Autodesk Inventor part; units mm, degrees
sketch "Sketch1" plane through (0, 0, 0) normal (0, 0, 1) x (1, 0, 0)
  line L0 (-10.75, -9.35) -> (10.75, -9.35)
  line L1 (10.75, -9.35) -> (10.75, 9.35)
  line L2 (10.75, 9.35) -> (-10.75, 9.35)
  line L3 (-10.75, 9.35) -> (-10.75, -9.35)
  line L4 (-10.75, -9.35) -> (10.75, 9.35) construction
  line L5 (10.75, -9.35) -> (-10.75, 9.35) construction
  point P0 (0, 0)
  dimension "d0" = 21.5
  dimension "d1" = 18.7
extrude "Extrusion1" add sketch "Sketch1" along normal mid plane 2.7
sketch "Sketch3" plane through (0, 0, 1.35) normal (0, 0, 1) x (1, 0, 0)
  line L0 (-8.75, -7.35) -> (8.75, -7.35)
  line L1 (8.75, -7.35) -> (8.75, 8.35)
  line L2 (8.75, 8.35) -> (-8.75, 8.35)
  line L3 (-8.75, 8.35) -> (-8.75, -7.35)
  line L4 (-8.75, -7.35) -> (8.75, 8.35) construction
  line L5 (8.75, -7.35) -> (-8.75, 8.35) construction
  line L6 (-10.75, -9.35) -> (10.75, -9.35)
  point P0 (0, 0.5)
  dimension "d8" = 17.5
  dimension "d47" = 2
  dimension "d61" = 15.7
extrude "Extrusion3" cut sketch "Sketch3" against normal blind 1.8
sketch "Sketch4" plane through (0, 0, 1.35) normal (0, 0, 1) x (1, 0, 0)
  line L0 (2.5, 5.884) -> (-2.5, 5.884)
  line L1 (-2.5, 5.884) -> (-2.5, 12.884)
  line L2 (-2.5, 12.884) -> (2.5, 12.884)
  line L3 (2.5, 12.884) -> (2.5, 5.884)
  line L4 (2.5, 5.884) -> (-2.5, 12.884) construction
  line L5 (-2.5, 5.884) -> (2.5, 12.884) construction
  point P0 (0, 0)
  point P1 (0, 9.384)
  dimension "d12" = 5
  dimension "d15" = 7
extrude "Extrusion4" cut sketch "Sketch4" against normal blind 3
sketch "Sketch7" plane through (-10.75, 0.5, 6.442) normal (1, 0, 0) x (0, -1, 0)
  line L0 (3.5, 6.442) -> (-2.5, 6.442)
  line L1 (-2.5, 6.442) -> (-2.5, 9.442)
  line L2 (-2.5, 9.442) -> (3.5, 9.442)
  line L3 (3.5, 9.442) -> (3.5, 6.442)
  line L4 (3.5, 6.442) -> (-2.5, 9.442) construction
  line L5 (-2.5, 6.442) -> (3.5, 9.442) construction
  line L6 (0.5, -1.8884) -> (0.5, 11.3304)
  line L7 (-8.85, 7.792) -> (-8.85, 5.092)
  point P0 (0, 0)
  point P1 (0.5, 7.942)
  point P2 (0.5, 7.942)
  point P3 (0.5, -1.8884)
  point P4 (0.5, 11.3304)
  point P5 (-8.85, 6.442)
  dimension "d24" = 6
  dimension "d23" = 3
extrude "Extrusion7" [suppressed]
fillet "Fillet1" [suppressed]
fillet "Fillet2" [suppressed]
fillet "Fillet3" [suppressed]
fillet "Fillet4" [suppressed]
fillet "Fillet5" [suppressed]
fillet "Fillet6" radius 0.2 1 edges at (10.75, 0, -1.35)
fillet "Fillet7" [suppressed]
fillet "Fillet8" [suppressed]
fillet "Fillet9" [suppressed]
fillet "Fillet10" [suppressed]
fillet "Fillet11" [suppressed]
mirror "Mirror2" [suppressed]
sketch "InsertPoles_Sketch" plane through (0, 0, 1.35) normal (0, 0, 1) x (1, 0, 0)
  circle A0 centre (-9.75, -8.35) radius 0.55
  line L0 (-10.75, 9.35) -> (-10.75, -9.35)
  line L1 (-10.75, -9.35) -> (10.75, -9.35)
  circle A1 centre (-9.75, -4.35) radius 0.55
  circle A2 centre (-9.75, 4.35) radius 0.55
  circle A3 centre (-9.75, 8.35) radius 0.55
  circle A4 centre (-5.75, -8.35) radius 0.55
  line L2 (-2.5, 9.35) -> (-10.75, 9.35)
  point P0 (0, 0)
  point P1 (-8.75, 9.35)
  dimension "d39" = 1.1
  dimension "d40" = 1
  dimension "d41" = 1
  dimension "d42" = 1.1
  dimension "d43" = 1.1
  dimension "d44" = 1.1
  dimension "d45" = 1.1
  dimension "d48" = 4
  dimension "d49" = 1
  dimension "d50" = 1
  dimension "d51" = 4
  dimension "d52" = 4
extrude "InsertPoles_Extrude" cut sketch "InsertPoles_Sketch" against normal blind 3
mirror "MirrorInsertPoles" about plane through (0, 0, 0) normal (1, 0, 0) of "InsertPoles_Extrude"
sketch "RibbonCableCutout_Sketch" plane through (0, 0, 1.35) normal (0, 0, 1) x (1, 0, 0)
  line L0 (3, -7.0087) -> (-3, -7.0087)
  line L1 (-3, -7.0087) -> (-3, -9.0087)
  line L2 (-3, -9.0087) -> (3, -9.0087)
  line L3 (3, -9.0087) -> (3, -7.0087)
  line L4 (3, -7.0087) -> (-3, -9.0087) construction
  line L5 (-3, -7.0087) -> (3, -9.0087) construction
  line L6 (0, 13.09) -> (0, -13.09)
  point P0 (0, 0)
  point P1 (0, -8.0087)
  point P2 (0, -8.0087)
  dimension "d56" = 6
  dimension "d57" = 2
extrude "RibbonCableCutout_Extrude" [suppressed]
fillet "Fillet12" [suppressed]
sketch "Sketch11" plane through (-0.0016, -9.35, -6.4418) normal (0, -1, 0) x (1, 0, 0)
  line L0 (3.9693, 3.0494) -> (-4.0307, 3.0494)
  line L1 (-4.0307, 3.0494) -> (-4.0307, 10.0494)
  line L2 (-4.0307, 10.0494) -> (3.9693, 10.0494)
  line L3 (3.9693, 10.0494) -> (3.9693, 3.0494)
  line L4 (3.9693, 3.0494) -> (-4.0307, 10.0494) construction
  line L5 (-4.0307, 3.0494) -> (3.9693, 10.0494) construction
  point P0 (0, 0)
  point P1 (-0.0307, 6.5494)
  dimension "d63" = 8
  dimension "d62" = 7
extrude "Extrusion10" cut sketch "Sketch11" against normal blind 3
properties part number "Checkpoint10.2_BackCover"
Geometry: final body of the model. Coordinates: model frame, mm. A direction names the side the tool comes from. Round coordinates to 2 decimals unless told otherwise and drop trailing zeros. Order: outer loops, then holes, each group sorted by start corner. A loop starts at its lowest first (then second) coordinate and runs counter-clockwise, first axis right, second up. Notation, with made-up numbers: M -20,80 L -15,80 A13 ccw -15,85 Z; hole C 55,41 d9. An arc over 180 degrees is marked long. Use one line per item in the form item = value. Start each with the question number.
Q1. Mould query, pull axis Y, two halves, no side actions, for faces 1 (the face through (2.5, 8, -1)), 2 (the face through (0, -6.35, -1)), 3 (the face through (-6, 8.35, 0)). Classes: +Y half, -Y half, draft (parallel to the pull), parting line (faces both ways), or undercut.
Q2. Cut plane B-B (y = -4.35). Return loops of the section in (x, z).
Q3. Cut plane A-A (z = -0.2). Count the separate pieces of the cut face and the enclosed holes in it, and give its area (3 significant figures).
Q4. Cut plane D-D (y = -8.35). Return loops of the section in (x, z).
Q5. Material intervals for line 1 (Y direction, x = 9.75, z = 0.3); line 2 (Y direction, x = -5.75, z = 0.3); line 3 (X direction, y = 6, z = -0.15), sorted ascending. Write a range as [from, to].
Q6. Access query for faces 4 (the face through (8.75, 0, 0)), 5 (the face through (-2.5, 8, -1)), 6 (the face through (-10.3, -8.33, 0.02)). Directions: +Z, -Z, +X, -X, +Y, -Y. A direction counts if a zero-diameter tool reaches every point of the face in a straight line with its end or side. Return the directions, or none.
Q7. Cut plane C-C (x = -5.75). Return loops of the section in (y, z), and give its area (3 significant figures).
Q8. Pin query (flat end, axial travel): pin 1 Ø1 at (x, y) = (-9.75, 4.35) entering from -Z. Return the tip coordinate at first contact, or that it passes through.
Geometry results:
q1.face_1 = draft
q1.face_2 = -Y half
q1.face_3 = undercut
q2.outline = M -10.75,-1.35 L -10.3,-1.35 L -10.3,1.35 L -10.75,1.35 Z; M -9.2,-1.35 L 9.2,-1.35 L 9.2,1.35 L 8.75,1.35 L 8.75,-0.45 L -8.75,-0.45 L -8.75,1.35 L -9.2,1.35 Z; M 10.3,-1.35 L 10.55,-1.35 A0.2 ccw 10.75,-1.15 L 10.75,1.35 L 10.3,1.35 Z
q3.separate_pieces = 2
q3.enclosed_holes = 10
q3.area = 96.8 mm^2
q4.outline = M -10.75,-1.35 L -10.3,-1.35 L -10.3,1.35 L -10.75,1.35 Z; M -9.2,-1.35 L -6.3,-1.35 L -6.3,1.35 L -9.2,1.35 Z; M -5.2,-1.35 L -4.03,-1.35 L -4.03,1.35 L -5.2,1.35 Z; M 3.97,-1.35 L 5.2,-1.35 L 5.2,1.35 L 3.97,1.35 Z; M 6.3,-1.35 L 9.2,-1.35 L 9.2,1.35 L 6.3,1.35 Z; M 10.3,-1.35 L 10.55,-1.35 A0.2 ccw 10.75,-1.15 L 10.75,1.35 L 10.3,1.35 Z
q5.line_1 = [-9.35, -8.9], [-7.8, -4.9], [-3.8, 3.8], [4.9, 7.8], [8.9, 9.35]
q5.line_2 = [-9.35, -8.9], [-7.8, -7.35], [8.35, 9.35]
q5.line_3 = [-10.75, -8.75], [8.75, 10.75]
q6.face_4 = +Z
q6.face_5 = +Z, -Z, +Y
q6.face_6 = +Z, -Z
q7.outline = M -9.35,-1.35 L -8.9,-1.35 L -8.9,1.35 L -9.35,1.35 Z; M -7.8,-1.35 L 9.35,-1.35 L 9.35,1.35 L 8.35,1.35 L 8.35,-0.45 L -7.35,-0.45 L -7.35,1.35 L -7.8,1.35 Z
q7.area = 19.3 mm^2
q8.pin_1 = through
